The model under review builds one solid part; all positions refer to its coordinate system, in mm. Face numbers are marked on the shaded views. A direction names the side the tool comes from. Coordinates: 2 decimals unless noted, no trailing zeros. Loops run counter-clockwise (first coordinate to the right, second up) from the corner with the lowest first, then second, coordinate; pieces in that order, holes last. Notation, with made-up numbers: M 67,-9 L 108,-9 A27 ccw 108,10 Z; hole C 80.5,-32 d7. An arc over 180 degrees is marked long. Write item = value, one per line. Start each with the question number.
Q1. We need section D-D on x = 4.5. Give the boundary of the cut face in (y, z).
Q2. We need section B-B on y = 7.5. Give the boundary of the cut face in (x, z), and give its area (3 significant figures).
Q3. For the marked faces 5, 6 and 7, list the 3-axis set-ups (+Z, -Z, +X, -X, +Y, -Y) from which the entire face can be reached by the end or side of a thin tool; tool diameter is ignored.
Q4. Mouldability with a two-part tool opening along Y and no side actions: class the marked faces 1, 2, 3 and 4 as released by +Y, released by -Y, zero draft, split by the parting line, or undercut.
Q5. We need section A-A on z = 1.75. Give the boundary of the cut face in (x, y), and give its area (3 significant figures).
Q6. Clearance check with flat-ended pins moving along their axes: pin 1 Ø6 at (x, y) = (-4, 3.5) entering from +Z; pin 2 Ø3.5 at (y, z) = (-9.5, 1.5) entering from -X; pin 3 Ø5.5 at (x, z) = (2, 12) entering from +Y. State where each tip first meets the part, or that it passes through.
Q7. Wall thickness on probe 1 along Y at (x, z) = (0, 7); probe 2 along Z at (x, y) = (6.5, -17); probe 3 along Z at (x, y) = (2.75, -5): over which ranges is each line inside the solid? List them lowest first.
Q8. We need section C-C on x = 0.5. Give the boundary of the cut face in (y, z), and give its area (3 significant figures).
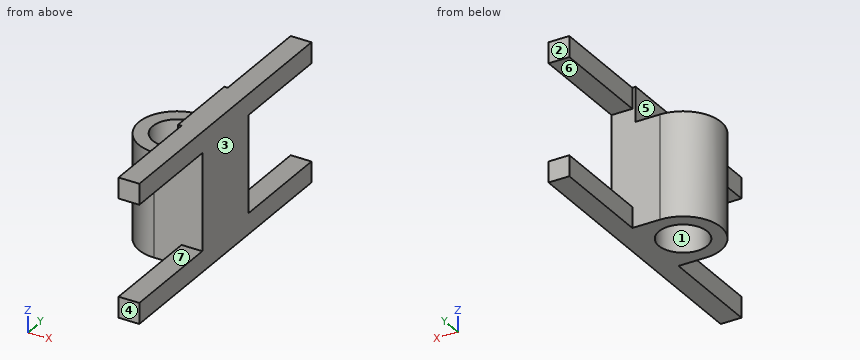
Autodesk Inventor part; units mm, degrees
ref_plane "YZ Plane" through (0, 0, 0) normal (1, 0, 0) x (0, 1, 0)
ref_plane "XZ Plane" through (0, 0, 0) normal (0, 1, 0) x (-1, 0, 0)
ref_plane "XY Plane" through (0, 0, 0) normal (0, 0, 1) x (1, 0, 0)
sketch "Sketch1" plane through (0, 0, 0) normal (0, 0, 1) x (1, 0, 0)
  circle A0 centre (0, 0) radius 5.5
  line L0 (0, 5.5) -> (11.9603, 5.5)
  line L1 (11.9603, 5.5) -> (11.9603, -5.5)
  line L2 (11.9603, -5.5) -> (0, -5.5)
  line L3 (0, -5.5) -> (0, 5.5)
  circle A1 centre (0, 0) radius 3.5
  dimension "d1" = 11
  dimension "d0" = 7
  dimension "d2" = 11
extrude "Extrusion1" add sketch "Sketch1" along normal blind 15 contours A0 L3 A1 | A0 L0 L1 L2 | L3 A1 A0 | A1 L3 picked at (0.9121, 0.7274)
sketch "Sketch2" plane through (0, 0, 15) normal (0, 0, 1) x (1, 0, 0)
  circle A0 centre (0, 0) radius 3.5
extrude "Extrusion2" cut sketch "Sketch2" against normal blind 15
sketch "Sketch3" plane through (0, 0, 15) normal (0, 0, 1) x (1, 0, 0)
  line L0 (11.9603, -5.5) -> (0, -5.5)
  line L1 (7, 5.5) -> (11.9603, 5.5)
  line L2 (11.9603, 5.5) -> (11.9603, -5.5)
  line L3 (11.9603, -5.5) -> (7, -5.5)
  line L4 (7, -5.5) -> (7, 5.5)
  line L5 (11.9603, -5.5) -> (11.9603, 5.5)
  line L6 (11.9603, 5.5) -> (0, 5.5)
  point P0 (0, 0)
  dimension "d7" = 7
  dimension "d8" = 0
  dimension "d9" = 0
extrude "Extrusion3" cut sketch "Sketch3" against normal blind 15
sketch "Sketch4" plane through (7, -5.5, 15) normal (1, 0, 0) x (0, 0, -1)
  point P0 (15, 5.5)
sketch "Sketch5" plane through (0, 0, 15) normal (0, 0, 1) x (1, 0, 0)
  point P0 (0, 0)
sketch "Sketch6" plane through (0, 0, 15) normal (0, 0, 1) x (1, 0, 0)
  line L0 (7, -5.5) -> (0, -5.5)
  line L1 (7, 5.5) -> (3.5, 5.5)
  line L2 (3.5, 5.5) -> (3.5, -5.5)
  line L3 (3.5, -5.5) -> (7, -5.5)
  line L4 (7, -5.5) -> (7, 5.5)
  point P0 (0, 0)
extrude "Extrusion4" add sketch "Sketch6" along normal blind 5
sketch "Sketch7" plane through (7, -5.5, 0) normal (1, 0, 0) x (0, 0, -1)
  line L0 (-3, -15) -> (0, -15)
  line L1 (0, -15) -> (0, 26)
  line L2 (0, 26) -> (-3, 26)
  line L3 (-3, 26) -> (-3, -15)
  line L4 (-20, -15) -> (-17, -15)
  line L5 (-17, -15) -> (-17, 26)
  line L6 (-17, 26) -> (-20, 26)
  line L7 (-20, 26) -> (-20, -15)
  line L8 (-20, 0) -> (-20, 11)
  line L9 (0, 0) -> (-20, 0)
  line L10 (-20, 11) -> (0, 11)
  point P0 (0, 5.5)
  dimension "d14" = 3
  dimension "d15" = 20
  dimension "d16" = 3
  dimension "d17" = 0
  dimension "d18" = 15
  dimension "d19" = 15
  dimension "d20" = 41
extrude "Extrusion5" add sketch "Sketch7" against normal blind 3 contours L3 L9 L1 L0 | L3 L10 L1 L9 | L3 L2 L1 L10 | L9 L7 L10 L5 | L5 L4 L7 L9 | L10 L7 L6 L5
properties part number "Slider"
Returned:
q1.outline = M -20.5,0 L 20.5,0 L 20.5,3 L 5.5,3 L 5.5,17 L 20.5,17 L 20.5,20 L -20.5,20 L -20.5,17 L -5.5,17 L -5.5,3 L -20.5,3 Z
q2.outline = M 4,0 L 7,0 L 7,3 L 4,3 Z; M 4,17 L 7,17 L 7,20 L 4,20 Z
q2.area = 18.0 mm^2
q3.face_5 = +Z, -X, +Y, -Y
q3.face_6 = +X, -X, +Y
q3.face_7 = +X, -X, -Y
q4.face_1 = undercut
q4.face_2 = released by +Y
q4.face_3 = zero draft
q4.face_4 = released by -Y
q5.outline = M 0,-5.5 L 4,-5.5 L 4,-20.5 L 7,-20.5 L 7,20.5 L 4,20.5 L 4,5.5 L 0,5.5 A5.5 ccw Z; hole C 0,0 d7
q5.area = 176 mm^2
q6.pin_1 = 15
q6.pin_2 = 4
q6.pin_3 = 5.5
q7.probe_1 = -5.5 to -3.5, 3.5 to 5.5
q7.probe_2 = 0 to 3, 17 to 20
q7.probe_3 = 0 to 15
q8.outline = M -5.5,0 L -3.46,0 L -3.46,15 L -5.5,15 Z; M 3.46,0 L 5.5,0 L 5.5,15 L 3.46,15 Z
q8.area = 61.1 mm^2
